Build history of the part. All positions in model axes, mm. A direction names the side the tool comes from. Round coordinates to 2 decimals unless told otherwise and drop trailing zeros. Write each loop counter-clockwise with the first axis right and the second up, starting at its lowest first coordinate (ties: lowest second). Pieces come first, ordered by that corner, then holes. Notation, with made-up numbers: (-32, -19.5) - (3, -19.5) arc R24 ccw to (3, 12.5) - close; hole circle Ø2 at (-17, 37). An arc over 180 degrees is marked (long way). One line per question, with ' | ' between items.
from build123d import *

# Parameters (mm, degrees)
BOSS_EXTRUDE1_DEPTH = 50.8
SKETCH3_R           = 4.9022
CUT_EXTRUDE1_DEPTH  = 50.8
SKETCH4_R           = 1.4732
CUT_EXTRUDE2_DEPTH  = 50.8
FILLET1_R           = 2.54


with BuildPart() as part:
    # Sketch2 → Boss-Extrude1 (new body)
    with BuildSketch(Plane(origin=(0, 0, 0), x_dir=(0, 0, -1), z_dir=(1, 0, 0))):
        Polygon((0, 0), (31.75, 0), (31.75, 31.75), (26.924, 31.75), (26.924, 4.826), (0, 4.826), align=None)
    extrude(amount=-BOSS_EXTRUDE1_DEPTH)

    # Sketch3 → Cut-Extrude1 (cut)
    with BuildSketch(Plane.XY.offset(-26.924)):
        with Locations((-38.1, 19.05)):
            Circle(SKETCH3_R)
        with Locations((-12.7, 19.05)):
            Circle(SKETCH3_R)
    extrude(amount=-CUT_EXTRUDE1_DEPTH, mode=Mode.SUBTRACT)

    # Sketch4 → Cut-Extrude2 (cut)
    with BuildSketch(Plane(origin=(0, 4.826, 0), x_dir=(1, 0, 0), z_dir=(0, 1, 0))):
        with Locations((-38.1, 12.7)):
            Circle(SKETCH4_R)
        with Locations((-12.7, 12.7)):
            Circle(SKETCH4_R)
    extrude(amount=-CUT_EXTRUDE2_DEPTH, mode=Mode.SUBTRACT)

    # Fillet1
    fillet1_edges = [part.edges().sort_by_distance(p)[0] for p in [
        (-25.4, 4.826, 0),
        (-25.4, 31.75, -26.924),
    ]]
    fillet(fillet1_edges, radius=FILLET1_R)


solid = part.part
Q1. Saw through at B-B, the plane y = 18. List the corners of the cut face in (x, z), then the cut area to 3 significant figures.
Found:
outline: (-50.8, -31.75) - (-42.89, -31.75) - (-42.89, -26.92) - (-50.8, -26.92) - close; (-33.31, -31.75) - (-17.49, -31.75) - (-17.49, -26.92) - (-33.31, -26.92) - close; (-7.91, -31.75) - (0, -31.75) - (0, -26.92) - (-7.91, -26.92) - close | area: 153 mm^2
Q2. Saw through at D-D, the plane x = -20.5. List the corners of the cut face in (y, z), then the cut area to 3 significant figures.
Found:
outline: (0, -31.75) - (31.75, -31.75) - (31.75, -29.46) arc R2.54 ccw to (29.21, -26.92) - (4.83, -26.92) - (4.83, -2.54) arc R2.54 ccw to (2.29, 0) - (0, 0) - close | area: 280 mm^2
Q3. Pull direction X, two halves, no side cores. Call faces 1 (the flat face through (-50.8, 10, -28)), 2 (the flat face through (-25, 4.826, -15)), 3 (the cylindrical face through (-38.42, 2.45, -11.26)): +X half, -X half, draft (parallel to the pull), parting line (faces both ways), or undercut.
Found:
face 1: -X half | face 2: draft | face 3: undercut
Q4. Saw through at C-C, the plane z = -12.7. List the corners of the cut face in (x, y).
Found:
outline: (-50.8, 0) - (-39.57, 0) - (-39.57, 4.83) - (-50.8, 4.83) - close; (-36.63, 0) - (-14.17, 0) - (-14.17, 4.83) - (-36.63, 4.83) - close; (-11.23, 0) - (0, 0) - (0, 4.83) - (-11.23, 4.83) - close
Q5. Drop flat-ended pins along their axis: pin 1 (4.5 mm diameter, centred on x = -38.1, z = -12.7, fed in from -Y); pin 2 (4 mm diameter, centred on x = -24, y = 26, fed in from +Z); pin 3 (1.5 mm diameter, centred on x = -41, z = -25, fed in from +Y). Give the stop position or say it passes through.
Found:
pin 1: y = 0 | pin 2: z = -26.92 | pin 3: y = 4.83
Q6. Saw through at A-A, the plane x = -12.7. List the corners of the cut face in (y, z), then the cut area to 3 significant figures.
Found:
outline: (0, -31.75) - (14.15, -31.75) - (14.15, -26.92) - (4.83, -26.92) - (4.83, -14.17) - (0, -14.17) - close; (0, -11.23) - (4.83, -11.23) - (4.83, -2.54) arc R2.54 ccw to (2.29, 0) - (0, 0) - close; (23.95, -31.75) - (31.75, -31.75) - (31.75, -29.46) arc R2.54 ccw to (29.21, -26.92) - (23.95, -26.92) - close | area: 219 mm^2
Q7. Drill centre lines: L1, parallel to X at y = 19, z = -28; L2, parallel to X at y = 3.7, z = -12.7; L3, parallel to Z at x = -26, y = 26.5. Where is each one in solid material? Low to high. Write a range as from..to.
Found:
L1: -50.8..-43, -33.2..-17.6, -7.8..0 | L2: -50.8..-39.57, -36.63..-14.17, -11.23..0 | L3: -31.75..-26.92
Q8. Which spindle directions (+Z, -Z, +X, -X, +Y, -Y) get a long thin tool onto all of the face, cutting with end or side? Do faces 4 (the flat face through (-25, 17, -26.924)), 5 (the flat face through (-25, 1, 0)). Say none if no direction does.
Found:
face 4: +Z, +X, -X, +Y | face 5: +Z, +X, -X, +Y, -Y
